```python
from build123d import *

# Parameters (mm, degrees)
F0_W      = 61.9125
F0_H      = 55.5625
F1_DEPTH  = 19.05
F3_DEPTH  = 58.7375
F4_W      = 3.175
F4_H      = 49.2125
F5_DEPTH  = 15.875
F7_DEPTH  = 15.875
F9_DEPTH  = 15.875
F10_W     = 19.05
F10_H     = 15.875
F10_W_2   = 3.175
F11_DEPTH = 101.6
F12_R     = 6.35
F13_W     = 25.4
F13_H     = 5.1575573161
F14_DEPTH = 25.4
F16_DEPTH = 25.4
F17_W     = 39.6875
F17_H     = 3.175
F18_DEPTH = 1.5875
F19_R     = 0.396875
F20_DEPTH = 25.4


with BuildPart() as f1:
    # F0 (on Top) → F1 (new body)
    with BuildSketch(Plane.XY):
        with Locations((-30.95625, 27.78125)):
            Rectangle(F0_W, F0_H)
    extrude(amount=F1_DEPTH)

    # F2 (on face) → F3 (cut)
    with BuildSketch(Plane.YZ):
        Polygon((27.78125, 15.875), (3.175, 15.875), (3.175, 0), (52.3875, 0), (52.3875, 15.875), align=None)
    extrude(amount=-F3_DEPTH, mode=Mode.SUBTRACT)

    # F4 (on face) → F5 (join)
    with BuildSketch(Plane(origin=(0, 0, 15.875), x_dir=(1, 0, 0), z_dir=(0, 0, -1))):
        with Locations((-1.5875, -27.78125)):
            Rectangle(F4_W, F4_H)
    extrude(amount=F5_DEPTH)

    # F6 (on face) → F7 (join)
    with BuildSketch(Plane(origin=(0, 0, 0), x_dir=(1, 0, 0), z_dir=(0, 0, -1))):
        Polygon((-61.9125, -3.175), (-58.7375, -3.175), (-3.175, -3.175), (0, -3.175), (0, 0), (-61.9125, 0), align=None)
    extrude(amount=F7_DEPTH)

    # F8 (on face) → F9 (join)
    with BuildSketch(Plane(origin=(0, 0, 0), x_dir=(1, 0, 0), z_dir=(0, 0, -1))):
        Polygon((-3.175, -52.3875), (-58.7375, -52.3875), (-61.9125, -52.3875), (-61.9125, -55.5625), (0, -55.5625), (0, -52.3875), align=None)
    extrude(amount=F9_DEPTH)

    # F10 (on face) → F11 (cut)
    with BuildSketch(Plane.XZ):
        with Locations((-52.3875, -7.9375)):
            Rectangle(F10_W, F10_H)
        with Locations((-1.5875, -7.9375)):
            Rectangle(F10_W_2, F10_H)
    extrude(amount=-F11_DEPTH, mode=Mode.SUBTRACT)

    # F12
    f12_edges = [f1.edges().sort_by_distance(p)[0] for p in [
        (-61.9125, 0, 9.525),
        (-30.95625, 0, 19.05),
        (-61.9125, 27.78125, 19.05),
        (0, 0, 9.525),
        (0, 27.78125, 19.05),
        (0, 55.5625, 9.525),
        (-61.9125, 55.5625, 9.525),
        (-30.95625, 55.5625, 19.05),
    ]]
    fillet(f12_edges, radius=F12_R)

    # F13 (on face) → F14 (cut)
    with BuildSketch(Plane.YZ):
        with Locations((27.78125, 2.5787786581)):
            Rectangle(F13_W, F13_H)
    extrude(amount=-F14_DEPTH, mode=Mode.SUBTRACT)

    # F15 (on face) → F16 (cut)
    with BuildSketch(Plane(origin=(0, 0, 15.875), x_dir=(1, 0, 0), z_dir=(0, 0, -1))):
        Polygon((-40.3606608115, -6.35), (-46.7106608115, -6.35), (-53.0606608115, -6.35), (-53.0606608115, -7.9375), (-40.3606608115, -7.9375), align=None)
        Polygon((-40.3606608115, -47.625), (-53.0606608115, -47.625), (-53.0606608115, -49.2125), (-46.7106608115, -49.2125), (-40.3606608115, -49.2125), align=None)
    extrude(amount=-F16_DEPTH, mode=Mode.SUBTRACT)

    # F17 (on face) → F18 (join)
    with BuildSketch(Plane.XZ.offset(-52.3875)):
        with Locations((-23.01875, -14.2875)):
            Rectangle(F17_W, F17_H)
    extrude(amount=F18_DEPTH)

    # F19 (on face) → F20 (cut)
    with BuildSketch(Plane.XY.offset(19.05)):
        with BuildLine():
            Line((-36.4952536137, 24.4581068784), (-36.0983786137, 24.4581068784))
            ThreePointArc((-36.0983786137, 24.4581068784), (-36.7758866175, 24.7387398822), (-36.4952536137, 24.0612318784))
            Line((-36.4952536137, 24.0612318784), (-36.4952536137, 24.4581068784))
        make_face()
        with BuildLine():
            ThreePointArc((-36.4952536137, 24.0612318784), (-36.2146206099, 24.1774738746), (-36.0983786137, 24.4581068784))
            Line((-36.0983786137, 24.4581068784), (-36.4952536137, 24.4581068784))
            Line((-36.4952536137, 24.4581068784), (-36.4952536137, 24.0612318784))
        make_face()
        with Locations((-34.4823842707, 25.6202375354)):
            Circle(F19_R)
        with Locations((-32.1581229567, 25.6202375354)):
            Circle(F19_R)
        with Locations((-30.1452536137, 24.4581068784)):
            Circle(F19_R)
        with Locations((-28.9831229567, 22.4452375354)):
            Circle(F19_R)
        with Locations((-28.9831229567, 20.1209762214)):
            Circle(F19_R)
        with Locations((-30.1452536137, 18.1081068784)):
            Circle(F19_R)
        with Locations((-32.1581229567, 16.9459762214)):
            Circle(F19_R)
        with Locations((-32.3391246566, 18.2635024392)):
            Circle(F19_R)
        with Locations((-30.7516246566, 19.4168887024)):
            Circle(F19_R)
        with BuildLine():
            ThreePointArc((-30.5421286137, 21.2831068784), (-30.1452536137, 20.8862318784), (-29.7483786137, 21.2831068784))
            Line((-29.7483786137, 21.2831068784), (-30.5421286137, 21.2831068784))
        make_face()
        with Locations((-31.5532411462, 20.6476470681)):
            Circle(F19_R)
        with Locations((-32.5201250566, 19.5843024392)):
            Circle(F19_R)
        with BuildLine():
            ThreePointArc((-33.3202536137, 20.8862318784), (-33.0396206099, 21.0024738746), (-32.9233786137, 21.2831068784))
            Line((-32.9233786137, 21.2831068784), (-33.3202536137, 21.2831068784))
            Line((-33.3202536137, 21.2831068784), (-33.3202536137, 20.8862318784))
        make_face()
        with BuildLine():
            Line((-30.5421286137, 21.2831068784), (-29.7483786137, 21.2831068784))
            ThreePointArc((-29.7483786137, 21.2831068784), (-30.1452536137, 21.6799818784), (-30.5421286137, 21.2831068784))
        make_face()
        with Locations((-31.6214491745, 22.0832354355)):
            Circle(F19_R)
        with BuildLine():
            Line((-33.3202536137, 21.2831068784), (-32.9233786137, 21.2831068784))
            ThreePointArc((-32.9233786137, 21.2831068784), (-33.0396206099, 21.5637398822), (-33.3202536137, 21.6799818784))
            Line((-33.3202536137, 21.6799818784), (-33.3202536137, 21.2831068784))
        make_face()
        with Locations((-32.6847938034, 23.0501193459)):
            Circle(F19_R)
        with Locations((-32.3391246566, 24.3027113176)):
            Circle(F19_R)
        with Locations((-30.7516246566, 23.1493250544)):
            Circle(F19_R)
        with BuildLine():
            Line((-34.1203821709, 22.9819113176), (-33.7235071709, 22.9819113176))
            ThreePointArc((-33.7235071709, 22.9819113176), (-34.4010151746, 23.2625443214), (-34.1203821709, 22.5850363176))
            Line((-34.1203821709, 22.5850363176), (-34.1203821709, 22.9819113176))
        make_face()
        with BuildLine():
            ThreePointArc((-34.1203821709, 22.5850363176), (-33.8397491671, 22.7012783139), (-33.7235071709, 22.9819113176))
            Line((-33.7235071709, 22.9819113176), (-34.1203821709, 22.9819113176))
            Line((-34.1203821709, 22.9819113176), (-34.1203821709, 22.5850363176))
        make_face()
        with BuildLine():
            ThreePointArc((-33.9045075709, 24.3027113176), (-33.9125101011, 24.3820080254), (-33.9361949679, 24.4581068784))
            Line((-33.9361949679, 24.4581068784), (-34.6665701738, 24.4581068784))
            ThreePointArc((-34.6665701738, 24.4581068784), (-34.3806792786, 23.9138388478), (-33.9045075709, 24.3027113176))
        make_face()
        with BuildLine():
            Line((-34.6665701738, 24.4581068784), (-33.9361949679, 24.4581068784))
            ThreePointArc((-33.9361949679, 24.4581068784), (-34.3013825709, 24.6995863176), (-34.6665701738, 24.4581068784))
        make_face()
        with Locations((-35.8888825709, 23.1493250544)):
            Circle(F19_R)
        with Locations((-35.0872660812, 21.9185666887)):
            Circle(F19_R)
        with BuildLine():
            Line((-33.7171286137, 21.2831068784), (-33.3202536137, 21.2831068784))
            Line((-33.3202536137, 21.2831068784), (-33.3202536137, 21.6799818784))
            ThreePointArc((-33.3202536137, 21.6799818784), (-33.6008866175, 21.5637398822), (-33.7171286137, 21.2831068784))
        make_face()
        with BuildLine():
            Line((-36.4952536137, 21.2831068784), (-36.0983786137, 21.2831068784))
            ThreePointArc((-36.0983786137, 21.2831068784), (-36.2146206099, 21.5637398822), (-36.4952536137, 21.6799818784))
            Line((-36.4952536137, 21.6799818784), (-36.4952536137, 21.2831068784))
        make_face()
        with BuildLine():
            Line((-36.8921286137, 21.2831068784), (-36.4952536137, 21.2831068784))
            Line((-36.4952536137, 21.2831068784), (-36.4952536137, 21.6799818784))
            ThreePointArc((-36.4952536137, 21.6799818784), (-36.7758866175, 21.5637398822), (-36.8921286137, 21.2831068784))
        make_face()
        with Locations((-37.6573842707, 22.4452375354)):
            Circle(F19_R)
        with Locations((-37.6573842707, 20.1209762214)):
            Circle(F19_R)
        with BuildLine():
            ThreePointArc((-36.8921286137, 21.2831068784), (-36.4952536137, 20.8862318784), (-36.0983786137, 21.2831068784))
            Line((-36.0983786137, 21.2831068784), (-36.4952536137, 21.2831068784))
            Line((-36.4952536137, 21.2831068784), (-36.8921286137, 21.2831068784))
        make_face()
        with Locations((-35.0190580529, 20.4829783213)):
            Circle(F19_R)
        with Locations((-35.8888825709, 19.4168887024)):
            Circle(F19_R)
        with Locations((-36.4952536137, 18.1081068784)):
            Circle(F19_R)
        with Locations((-34.4823842707, 16.9459762214)):
            Circle(F19_R)
        with Locations((-34.3013825709, 18.2635024392)):
            Circle(F19_R)
        with Locations((-33.955713424, 19.5160944109)):
            Circle(F19_R)
        with BuildLine():
            ThreePointArc((-33.7171286137, 21.2831068784), (-33.6008866175, 21.0024738746), (-33.3202536137, 20.8862318784))
            Line((-33.3202536137, 20.8862318784), (-33.3202536137, 21.2831068784))
            Line((-33.3202536137, 21.2831068784), (-33.7171286137, 21.2831068784))
        make_face()
    extrude(amount=-F20_DEPTH, mode=Mode.SUBTRACT)


solid = f1.part
```
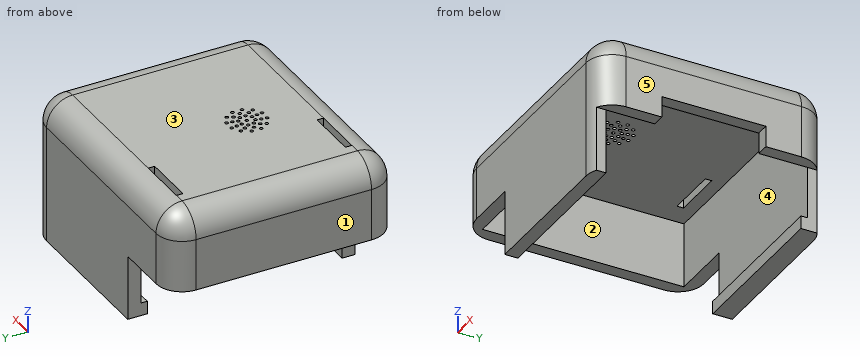
Build history of the part. All positions in model axes, mm. Face numbers are marked on the shaded views. A direction names the side the tool comes from. Round coordinates to 2 decimals unless told otherwise and drop trailing zeros. Write each question's results on one line, items separated by ' | '. Start each with the question number.
Item 1: Wall check: L1, parallel to X at y = 11.5, z = 12 (1 decimal); L2, parallel to Y at x = -12.5, z = 3.5 (1 decimal); L3, parallel to Z at x = -29, y = 25 (3 decimals). Give the ranges that are in metal, low to high. Write a range as [from, to].
Item 2: Drop flat-ended pins along their axis: P1, Ø1, axis at x = -1.5, z = 2, coming from the +Y side; P2, Ø1.7, axis at y = 49, z = 18, coming from the +X side; P3, Ø1.6, axis at x = -2, y = 50.5, coming from the -Z side; P4, Ø10, axis at y = 8.5, z = -10, coming from the -X side. Give the stop position or say it passes through.
Item 3: Saw through at B-B (x = -50.5). State how many separate pieces and enclosed holes the cut face has, and give its area (3 significant figures).
Item 4: Which spindle directions (+Z, -Z, +X, -X, +Y, -Y) get a long thin tool onto all of the face, cutting with end or side? Do the marked faces 1 and 2. Say none if no direction does.
Item 5: Mould opens along X. For the marked faces 3, 4 and 5 say: pulls with the +X half, pulls with the -X half, needs draft (parallel to the pull), parting line crosses it, or undercut.
Results are:
1) L1: x = [-61.9, -58.7], [-3.2, 0] | L2: y = [0, 3.2], [52.4, 55.6] | L3: z = [15.875, 19.05]
2) P1: stops at y = 53.84 | P2: stops at x = -1.82 | P3: stops at z = 0 | P4: passes through
3) separate pieces: 3 | enclosed holes: 0 | area: 250 mm²
4) face 1: +Z, -Z, -X, +Y, -Y | face 2: -Z
5) face 3: needs draft | face 4: undercut | face 5: pulls with the +X half
